Here's how the part is built. I have some questions about the finished solid (model axes, mm). A direction names the side the tool comes from. Give positions to 0.01 mm unless a question says otherwise; leave off trailing zeros. Write each loop counter-clockwise with the first axis right and the second up, starting at its lowest first coordinate (ties: lowest second). Pieces come first, ordered by that corner, then holes. Notation, with made-up numbers: M 7,-28 L 18,-28 A23 cw 18,-4 Z; hole C 51.5,57 d3. An arc over 180 degrees is marked long. Answer as CSV lines item,"result". Start each with the question number.
Q1. For pin 1 (3 mm diameter, centred on x = -1.5, y = -0.5, fed in from -Z); pin 2 (1.2 mm diameter, centred on x = 0, y = 0, fed in from +Z), each with a flat end and sliding along its axis, tell me the tip position at first contact or that it passes through.
Q2. Thinking about a two-plate mould opening in X: for faces 1 (the flat face through (1.1, 0, 0)), 2 (the cylindrical face through (-0.19, -0.87, -1.5)), 3 (the cylindrical face through (-0.22, 0.99, 7.33)), 4 (the flat face through (-2.54, 0, 5)), which applies, +X half, -X half, draft (parallel to the pull), parting line (faces both ways), or undercut?
Q3. Suppose I cut it at D-D (y = -1.4). Write out the boundary of the cut face in (x, z), then the cut area to 3 significant figures.
Q4. Suppose I cut it at A-A (x = 0). Write out the boundary of the cut face in (y, z).
Q5. On a 3-axis mill with a long thin cutter (end or side, diameter ignored), from which of +Z, -Z, +X, -X, +Y, -Y can I reach the whole of each face in a straight line? I mean faces 5 (the flat face through (0, 2.54, 5)), 6 (the flat face through (0, 0, 4.572)). Say none if no direction works.
Q6. If I drill on line 1 along Y through (x, z) = (0, 8.4); line 2 along Z through (x, y) = (-2.25, 1.8); line 3 along X through (y, z) = (-0.6, 6), over which ranges is the centre line in solid material (lowest first)?
Q7. Suppose I cut it at C-C (z = 5). Write out the boundary of the cut face in (x, y).
Autodesk Fusion 360 part; units mm, degrees
sketch "Sketch1" plane through (0, 0, 0) normal (0, 0, 1) x (1, 0, 0)
  circle A0 centre (0, 0) radius 1.016
  circle A1 centre (0, 0) radius 0.889
  line L0 (2.54, 2.54) -> (-2.54, 2.54)
  line L1 (-2.54, 2.54) -> (-2.54, -2.54)
  line L2 (-2.54, -2.54) -> (2.54, -2.54)
  line L3 (2.54, -2.54) -> (2.54, 2.54)
  line L4 (2.54, 2.54) -> (-2.54, -2.54) construction
  line L5 (-2.54, 2.54) -> (2.54, -2.54) construction
  dimension "d2" = 2.032
  dimension "d7" = 1.778
  dimension "d10" = 5.08
  dimension "d11" = 5.08
extrude "Extrude1" add sketch "Sketch1" along normal blind 10.16 contours L0 L1 L2 L3
extrude "Extrude2" add sketch "Sketch1" along normal blind 4.572 contours A0 | A1
extrude "Extrude3" add sketch "Sketch1" against normal blind 3.048 contours A1
Resolved:
1,pin 1,"z = -3.05"
1,pin 2,"z = 4.57"
2,face 1,"draft"
2,face 2,"parting line"
2,face 3,"undercut"
2,face 4,"-X half"
3,outline,"M -2.54,0 L 2.54,0 L 2.54,10.16 L -2.54,10.16 Z"
3,area,"51.6 mm^2"
4,outline,"M -2.54,0 L -0.89,0 L -0.89,-3.05 L 0.89,-3.05 L 0.89,0 L 2.54,0 L 2.54,10.16 L 1.02,10.16 L 1.02,4.57 L -1.02,4.57 L -1.02,10.16 L -2.54,10.16 Z"
5,face 5,"+Z, -Z, +X, -X, +Y"
5,face 6,"+Z"
6,line 1,"-2.54 to -1.02, 1.02 to 2.54"
6,line 2,"0 to 10.16"
6,line 3,"-2.54 to -0.82, 0.82 to 2.54"
7,outline,"M -2.54,-2.54 L 2.54,-2.54 L 2.54,2.54 L -2.54,2.54 Z; hole C 0,0 d2.03"
